Build history of the part. All positions in model axes, mm. Face numbers are marked on the shaded views. A direction names the side the tool comes from. Round coordinates to 2 decimals unless told otherwise and drop trailing zeros. Loops run counter-clockwise (first coordinate to the right, second up) from the corner with the lowest first, then second, coordinate; pieces in that order, holes last. Notation, with made-up numbers: (25, 75) - (60, 75) arc R16 cw to (60, 95) - close; hole circle Ø9 at (10, -13.75). An arc over 180 degrees is marked (long way). Use a Markdown table: item, result.
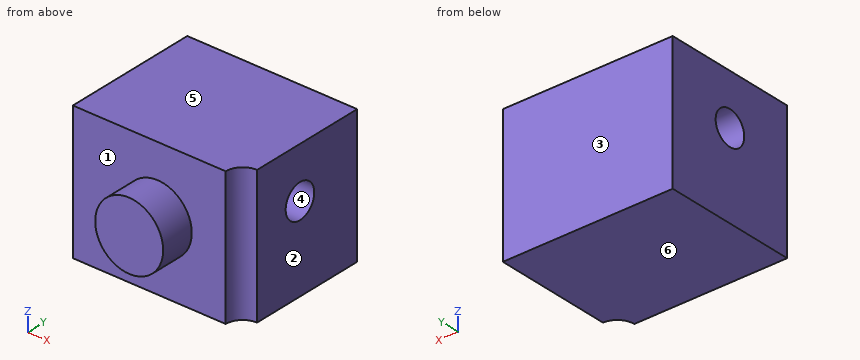
from build123d import *

# Parameters (mm, degrees)
F0_W     = 5
F0_H     = 4
F1_DEPTH = 4
F2_R     = 1
F3_DEPTH = 1
F5_DEPTH = 25
F6_R     = 0.5
F7_DEPTH = 5


with BuildPart() as f1:
    # F0 (on Top) → F1 (new body)
    with BuildSketch(Plane.XY):
        with Locations((2.5, 2)):
            Rectangle(F0_W, F0_H)
    extrude(amount=F1_DEPTH)

    # F2 (on face) → F3 (join)
    with BuildSketch(Plane.XZ):
        with Locations((2.5, 2)):
            Circle(F2_R)
    extrude(amount=F3_DEPTH)

    # F4 (on face) → F5 (cut)
    with BuildSketch(Plane.XY.offset(4)):
        with BuildLine():
            Line((5, 0), (5, 0.5))
            ThreePointArc((5, 0.5), (4.646447, 0.353553), (4.5, 0))
            Line((4.5, 0), (5, 0))
        make_face()
        with BuildLine():
            ThreePointArc((4.5, 0), (5, -0.5), (5.5, 0))
            ThreePointArc((5.5, 0), (5.353553, 0.353553), (5, 0.5))
            Line((5, 0.5), (5, 0))
            Line((5, 0), (4.5, 0))
        make_face()
    extrude(amount=-F5_DEPTH, mode=Mode.SUBTRACT)

    # F6 (on face) → F7 (cut)
    with BuildSketch(Plane.YZ.offset(5)):
        with Locations((2, 2.5)):
            Circle(F6_R)
    extrude(amount=-F7_DEPTH, mode=Mode.SUBTRACT)


solid = f1.part
Q1. Cut at B-B, the plane x = 1. List the corners of the cut face in (y, z), plus the area to 3 significant figures.
Results found:
| item | result |
|---|---|
| outline | (0, 0) - (4, 0) - (4, 4) - (0, 4) - close; hole circle Ø1 at (2, 2.5) |
| area | 15.2 mm2 |
Q2. Cut at D-D, the plane y = 2.3. List the corners of the cut face in (x, z).
Results found:
| item | result |
|---|---|
| outline | (0, 0) - (5, 0) - (5, 2.1) - (0, 2.1) - close; (0, 2.9) - (5, 2.9) - (5, 4) - (0, 4) - close |
Q3. Pull direction Z, two halves, no side cores. Call the marked faces 3, 4, 5 and 6: pulls with the +Z half, pulls with the -Z half, needs draft (parallel to the pull), parting line crosses it, or undercut.
Results found:
| item | result |
|---|---|
| face 3 | needs draft |
| face 4 | undercut |
| face 5 | pulls with the +Z half |
| face 6 | pulls with the -Z half |
Q4. Cut at C-C, the plane z = 2.5. List the corners of the cut face in (x, y), plus the area to 3 significant figures.
Results found:
| item | result |
|---|---|
| outline | (0, 0) - (1.63, 0) - (1.63, -1) - (3.37, -1) - (3.37, 0) - (4.5, 0) arc R0.5 cw to (5, 0.5) - (5, 1.5) - (0, 1.5) - close; (0, 2.5) - (5, 2.5) - (5, 4) - (0, 4) - close |
| area | 16.5 mm2 |
Q5. Which spindle directions (+Z, -Z, +X, -X, +Y, -Y) get a long thin tool onto all of the face, cutting with end or side? Do the marked faces 1 and 2. Say none if no direction does.
Results found:
| item | result |
|---|---|
| face 1 | -Y |
| face 2 | +Z, -Z, +X, +Y, -Y |
Q6. Drop a flat-ended pin along its axis: pin 1 (1.5 mm diameter, centred on x = 0.5, z = 0.5, fed in from -Y). Give the stop position or say it passes through.
Results found:
| item | result |
|---|---|
| pin 1 | stops at y = 0 |
Q7. Cut at A-A, the plane y = 1.6. List the corners of the cut face in (x, z).
Results found:
| item | result |
|---|---|
| outline | (0, 0) - (5, 0) - (5, 2.2) - (0, 2.2) - close; (0, 2.8) - (5, 2.8) - (5, 4) - (0, 4) - close |
Q8. Probe line 1 (Z direction, x = 3.05, y = 2); line 2 (Y direction, x = 1.8, z = 0.95); line 3 (Z direction, x = 0.3, y = 1.6). List the from-to ranges inside material, lowest first.
Results found:
| item | result |
|---|---|
| line 1 | z = 0 to 2, 3 to 4 |
| line 2 | y = 0 to 4 |
| line 3 | z = 0 to 2.2, 2.8 to 4 |
